The model under review builds one solid part; all positions refer to its coordinate system, in mm. Face numbers are marked on the shaded views. A direction names the side the tool comes from. Coordinates: 2 decimals unless noted, no trailing zeros. Loops run counter-clockwise (first coordinate to the right, second up) from the corner with the lowest first, then second, coordinate; pieces in that order, holes last. Notation, with made-up numbers: (4, 19) - (34, 19) arc R30 cw to (34, 55) - close; hole circle Ø1 at (-21, 10). An arc over 180 degrees is marked (long way). One line per item, written item: value. Start each with the question number.
1. To check wall thickness, follow line 1 (X direction, y = -16, z = 5.25); line 2 (Y direction, x = 0.5, z = 10.5); line 3 (Y direction, x = 13.5, z = 5.25). State the ranges of each line that lie inside material, in increasing order.
2. We need section C-C, the plane x = -20. Give the boundary of the cut face in (y, z).
3. We need section A-A, the plane z = 22.5. Give the boundary of the cut face in (x, y), then the cut area to 3 significant figures.
4. Insertion check: P1, Ø9.5, axis at x = -14.5, y = 7.5, coming from the +Z side; P2, Ø1, axis at x = -8.5, y = -1.5, coming from the -Z side. Each pin has a flat end and moves straight along its axis. Give the tip position at first contact, or say it passes through.
5. Mouldability with a two-part tool opening along Y and no side actions: class the marked faces 1, 2, 3 and 4 as +Y half, -Y half, draft (parallel to the pull), parting line (faces both ways), or undercut.
6. We need section B-B, the plane y = -11. Give the boundary of the cut face in (x, z).
7. We need section D-D, the plane x = 5. Give the boundary of the cut face in (y, z).
8. For the marked faces 5 and 6, list the 3-axis set-ups (+Z, -Z, +X, -X, +Y, -Y) from which the entire face can be reached by the end or side of a thin tool; tool diameter is ignored.
from build123d import *

# Parameters (mm, degrees)
F0_W     = 57
F0_H     = 71
F1_DEPTH = 30
F2_W     = 31
F2_H     = 45
F2_W_2   = 15
F2_H_2   = 39
F3_DEPTH = 25
F4_R     = 7
F5_R     = 3


with BuildPart() as f1:
    # F0 (on Top) → F1 (new body)
    with BuildSketch(Plane.XY):
        Rectangle(F0_W, F0_H)
    extrude(amount=F1_DEPTH)

    # F2 (on face) → F3 (cut)
    with BuildSketch(Plane.XY.offset(30)):
        with Locations((-9.34, -0.5)):
            Rectangle(F2_W, F2_H)
        with Locations((17.33, 0)):
            Rectangle(F2_W_2, F2_H_2)
    extrude(amount=-F3_DEPTH, mode=Mode.SUBTRACT)

    # F4
    f4_edges = [f1.edges().sort_by_distance(p)[0] for p in [
        (28.5, 35.5, 15),
        (28.5, -35.5, 15),
        (-28.5, -35.5, 15),
        (-28.5, 35.5, 15),
    ]]
    fillet(f4_edges, radius=F4_R)

    # F5
    f5_edges = [f1.edges().sort_by_distance(p)[0] for p in [
        (24.83, 19.5, 17.5),
        (24.83, -19.5, 17.5),
        (6.16, -23, 17.5),
        (6.16, 22, 17.5),
        (-24.84, 22, 17.5),
        (9.83, 19.5, 17.5),
        (-24.84, -23, 17.5),
        (9.83, -19.5, 17.5),
    ]]
    fillet(f5_edges, radius=F5_R)


solid = f1.part
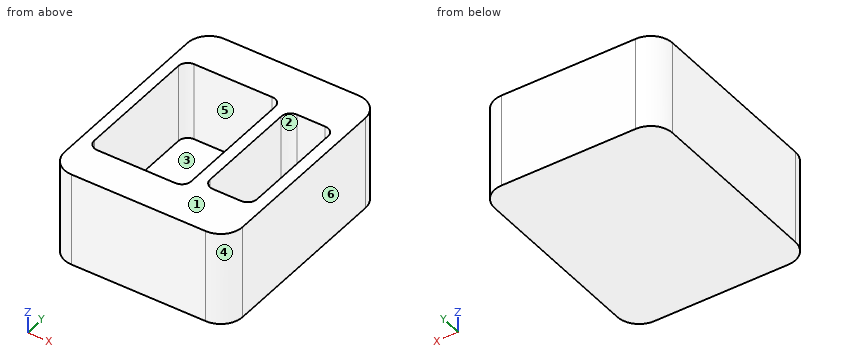
Findings below:
1. line 1: -28.5 to -24.84, 6.16 to 9.83, 24.83 to 28.5
1. line 2: -35.5 to -23, 22 to 35.5
1. line 3: -35.5 to -19.5, 19.5 to 35.5
2. outline: (-35.5, 0) - (35.5, 0) - (35.5, 30) - (22, 30) - (22, 5) - (-23, 5) - (-23, 30) - (-35.5, 30) - close
3. outline: (-28.5, -28.5) arc R7 ccw to (-21.5, -35.5) - (21.5, -35.5) arc R7 ccw to (28.5, -28.5) - (28.5, 28.5) arc R7 ccw to (21.5, 35.5) - (-21.5, 35.5) arc R7 ccw to (-28.5, 28.5) - close; hole (-24.84, -20) arc R3 ccw to (-21.84, -23) - (3.16, -23) arc R3 ccw to (6.16, -20) - (6.16, 19) arc R3 ccw to (3.16, 22) - (-21.84, 22) arc R3 ccw to (-24.84, 19) - close; hole (9.83, -16.5) arc R3 ccw to (12.83, -19.5) - (21.83, -19.5) arc R3 ccw to (24.83, -16.5) - (24.83, 16.5) arc R3 ccw to (21.83, 19.5) - (12.83, 19.5) arc R3 ccw to (9.83, 16.5) - close
3. area: 2,040 mm2
4. P1: z = 5
4. P2: z = 0
5. face 1: draft
5. face 2: undercut
5. face 3: undercut
5. face 4: -Y half
6. outline: (-28.5, 0) - (28.5, 0) - (28.5, 30) - (24.83, 30) - (24.83, 5) - (9.83, 5) - (9.83, 30) - (6.16, 30) - (6.16, 5) - (-24.84, 5) - (-24.84, 30) - (-28.5, 30) - close
7. outline: (-35.5, 0) - (35.5, 0) - (35.5, 30) - (21.37, 30) - (21.37, 5) - (-22.37, 5) - (-22.37, 30) - (-35.5, 30) - close
8. face 5: +Z
8. face 6: +Z, -Z, +X, +Y, -Y
